Build history of the part. All positions in model axes, mm. A direction names the side the tool comes from. Give positions to 0.01 mm unless a question says otherwise; leave off trailing zeros. Order: outer loops, then holes, each group sorted by start corner. A loop starts at its lowest first (then second) coordinate and runs counter-clockwise, first axis right, second up. Notation, with made-up numbers: (-17.75, -31) - (-8.75, -31) arc R22 ccw to (-8.75, -10) - close; hole circle Ø8 at (-15, -15). An arc over 180 degrees is marked (long way). Write each question's results on one line, items separated by ' | '. Start each with the question number.
1) Cut at D-D on x = -2. List the corners of the cut face in (y, z) (3 decimals), plus the area to 3 significant figures.
2) Tool access for faces 4 (the face through (2, 0, 0)), 5 (the face through (-0.34, 1.55, 6.14)), 6 (the face through (5, 0, 3.81)), 7 (the face through (-1.695, 4.296, 2.191)), 8 (the face through (0, 0, 7.874)): list every direction of +Z, -Z, +X, -X, +Y, -Y with a clear straight run to the whole face (end or side of a thin tool).
3) Drill centre lines: line 1 along Y through (x, z) = (-1.5, 3.25); line 2 along Z through (x, y) = (2, -1.75) (3 decimals); line 3 along Y through (x, z) = (3.5, 3.5). Where is each one in solid material? Low to high. Write a range as from..to.
4) Two-plate mould, pull along Y, no slides. Class faces 1 (the face through (6.982, -0.195, 2.191)), 2 (the face through (-1.661, -4.237, 2.191)), 3 (the face through (2, 0, 4.445)): +Y half, -Y half, draft (parallel to the pull), parting line (faces both ways), or undercut.
5) Cut at B-B on y = 0. List the corners of the cut face in (x, z) (1 decimal), plus the area to 3 significant figures.
6) Cut at A-A on x = 0. List the corners of the cut face in (y, z) (1 decimal).
7) Cut at C-C on z = 2.5. List the corners of the cut face in (x, y) (1 decimal), plus the area to 3 significant figures.
8) Drop flat-ended pins along their axis: pin 1 Ø1.6 at (x, y) = (5, 0) entering from -Z; pin 2 Ø2 at (x, y) = (0, 4) entering from +Z (3 decimals). Give the stop position or say it passes through.
from build123d import *

# Parameters (mm, degrees)
F0_R     = 1.5875
F0_R_2   = 1.6002
F1_DEPTH = 4.445
F2_R     = 1.5875
F3_DEPTH = 7.874
F4_R     = 1.6002
F5_DEPTH = 0.635


with BuildPart() as f1:
    # F0 (on Top) → F1 (new body)
    with BuildSketch(Plane.XY):
        with BuildLine():
            Line((-0.469262, -2.172395), (-2.887193, -6.360373))
            ThreePointArc((-2.887193, -6.360373), (6.985, 0), (-2.887193, 6.360373))
            Line((-2.887193, 6.360373), (-0.469262, 2.172395))
            ThreePointArc((-0.469262, 2.172395), (-2.2225, 0), (-0.469262, -2.172395))
        make_face()
        Circle(F0_R, mode=Mode.SUBTRACT)
        with Locations((4.826, 0)):
            Circle(F0_R_2, mode=Mode.SUBTRACT)
    extrude(amount=F1_DEPTH)

    # F2 (on face) → F3 (join)
    with BuildSketch(Plane(origin=(0, 0, 0), x_dir=(1, 0, 0), z_dir=(0, 0, -1))):
        Circle(F2_R)
    extrude(amount=-F3_DEPTH)

    # F4 (on face) → F5 (join)
    with BuildSketch(Plane.XY.offset(4.445)):
        with Locations((4.826, 0)):
            Circle(F4_R)
    extrude(amount=-F5_DEPTH)


solid = f1.part
Results:
1) outline: (-6.693, 0) - (-4.824, 0) - (-4.824, 4.445) - (-6.693, 4.445) - close; (-0.969, 0) - (0.969, 0) - (0.969, 4.445) - (-0.969, 4.445) - close; (4.824, 0) - (6.693, 0) - (6.693, 4.445) - (4.824, 4.445) - close | area: 25.2 mm^2
2) face 4: -Z, +X, -X, +Y, -Y | face 5: +Z | face 6: -Z | face 7: +Z, -Z, -X | face 8: +Z, +X, -X, +Y, -Y
3) line 1: -6.82..-3.96, -1.64..1.64, 3.96..6.82 | line 2: 0..4.445 | line 3: -6.04..-0.9, 0.9..6.04
4) face 1: parting line | face 2: undercut | face 3: draft
5) outline: (-2.2, 0) - (3.2, 0) - (3.2, 3.8) - (6.4, 3.8) - (6.4, 0) - (7, 0) - (7, 4.4) - (1.6, 4.4) - (1.6, 7.9) - (-1.6, 7.9) - (-1.6, 4.4) - (-2.2, 4.4) - close | area: 39.6 mm^2
6) outline: (-7, 0) - (7, 0) - (7, 4.4) - (1.6, 4.4) - (1.6, 7.9) - (-1.6, 7.9) - (-1.6, 4.4) - (-7, 4.4) - close
7) outline: (-2.9, -6.4) arc R7 ccw (long way) to (-2.9, 6.4) - (-0.5, 2.2) arc R2.2 ccw to (-0.5, -2.2) - close; hole circle Ø3.2 at (4.8, 0) | area: 92.8 mm^2
8) pin 1: z = 3.81 | pin 2: z = 4.445
